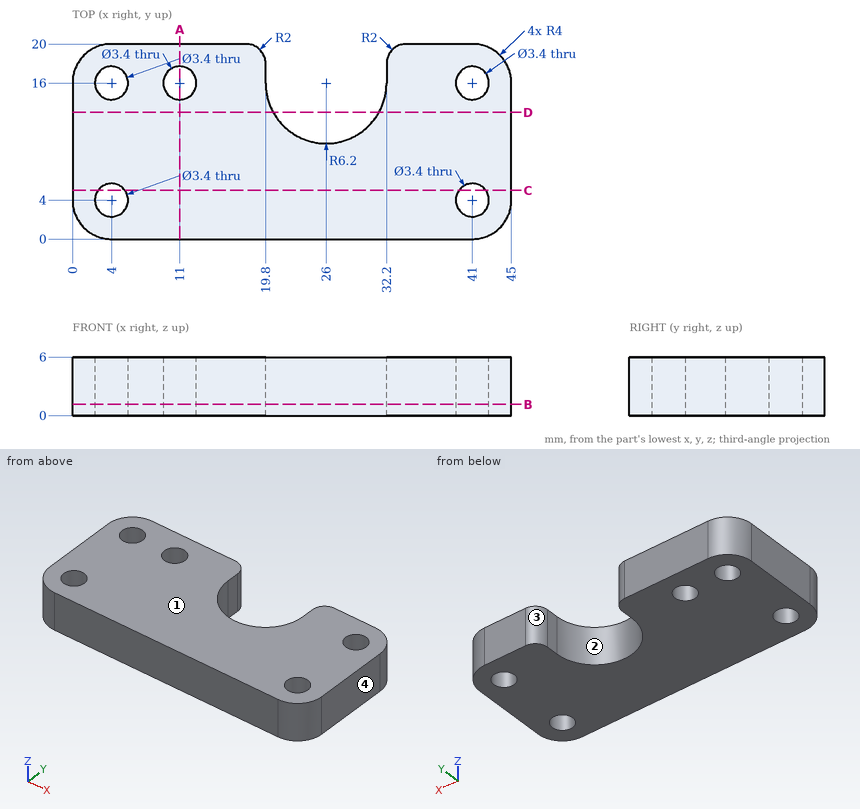
Design review of the part shown in the three views and the two pictorial views. Dimensions are in mm from the part's minimum x, y and z. Give positions to 0.01 mm unless a question says otherwise; leave off trailing zeros. Loops run counter-clockwise (first coordinate to the right, second up) from the corner with the lowest first, then second, coordinate; pieces in that order, holes last. Notation, with made-up numbers: (27.5, 13) - (67.5, 13) arc R20 ccw to (67.5, 45) - close; hole circle Ø11 at (43, 34.25). An arc over 180 degrees is marked (long way). Answer as a JSON object with one key per item and string values.
Q1. Add section A-A on x = 11. State the section outline as (y, z) points, plus the area to 3 significant figures.
Worked out:
{"outline": "(0, 0) - (14.3, 0) - (14.3, 6) - (0, 6) - close; (17.7, 0) - (20, 0) - (20, 6) - (17.7, 6) - close", "area": "99.6 mm^2"}
Q2. Add section B-B on z = 1.15. State the section outline as (x, y) points, plus the area to 3 significant figures.
Worked out:
{"outline": "(0, 4) arc R4 ccw to (4, 0) - (41, 0) arc R4 ccw to (45, 4) - (45, 16) arc R4 ccw to (41, 20) - (34.2, 20) arc R2 ccw to (32.2, 18) - (32.2, 16) arc R6.2 cw to (19.8, 16) - (19.8, 18) arc R2 ccw to (17.8, 20) - (4, 20) arc R4 ccw to (0, 16) - close; hole circle Ø3.4 at (4, 4); hole circle Ø3.4 at (4, 16); hole circle Ø3.4 at (11, 16); hole circle Ø3.4 at (41, 4); hole circle Ø3.4 at (41, 16)", "area": "729 mm^2"}
Q3. To check wall thickness, follow line 1 along Y through (x, z) = (4, 3.75); line 2 along X through (y, z) = (3.5, 4.1); line 3 along X through (y, z) = (17.25, 1.95). State the ranges of each line that lie inside material, in increasing order.
Worked out:
{"line 1": "y = 0 to 2.3, 5.7 to 14.3, 17.7 to 20", "line 2": "x = 0.03 to 2.38, 5.62 to 39.38, 42.62 to 44.97", "line 3": "x = 0.2 to 2.85, 5.15 to 9.85, 12.15 to 19.8, 32.2 to 39.85, 42.15 to 44.8"}
Q4. Mouldability with a two-part tool opening along X and no side actions: class the marked faces 1, 2, 3 and 4 as +X half, -X half, draft (parallel to the pull), parting line (faces both ways), or undercut.
Worked out:
{"face 1": "draft", "face 2": "undercut", "face 3": "undercut", "face 4": "+X half"}
Q5. Add section D-D on y = 13. State the section outline as (x, z) points.
Worked out:
{"outline": "(0, 0) - (20.57, 0) - (20.57, 6) - (0, 6) - close; (31.43, 0) - (45, 0) - (45, 6) - (31.43, 6) - close"}
Q6. Insertion check: pin 1 (0.6 mm diameter, centred on y = 16.5, z = 4, fed in from -X) (3 decimals); pin 2 (1.5 mm diameter, centred on x = 30.5, z = 2.5, fed in from +Y); pin 3 (3 mm diameter, centred on x = 41, y = 4, fed in from -Z); pin 4 (2 mm diameter, centred on x = 26, z = 3, fed in from +Y). Each pin has a flat end and moves straight along its axis. Give the tip position at first contact, or say it passes through.
Worked out:
{"pin 1": "stops at x = 0.005", "pin 2": "stops at y = 12.7", "pin 3": "passes through", "pin 4": "stops at y = 9.88"}
Q7. Add section C-C on y = 5. State the section outline as (x, z) points.
Worked out:
{"outline": "(0, 0) - (2.63, 0) - (2.63, 6) - (0, 6) - close; (5.37, 0) - (39.63, 0) - (39.63, 6) - (5.37, 6) - close; (42.37, 0) - (45, 0) - (45, 6) - (42.37, 6) - close"}
